from build123d import *

# Parameters (mm, degrees)
ESQUISSE1_W               = 60.5
ESQUISSE1_H               = 64
BOSS_EXTRU_1_DEPTH        = 30
ESQUISSE2_R               = 4.5
ENL_V_MAT_EXTRU_1_DEPTH   = 32
ENL_V_MAT_EXTRU_2_REACH   = 55.283
ESQUISSE4_W               = 51.1
ESQUISSE4_H               = 83.557669167
ESQUISSE5_R               = 10.5
ENL_V_MAT_EXTRU_3_DEPTH   = 2
ESQUISSE6_R               = 10
ENL_V_MAT_EXTRU_4_DEPTH   = 4.7
ESQUISSE7_W               = 47
ESQUISSE7_H               = 57
BOSS_EXTRU_2_DEPTH        = 30
ENL_V_MAT_EXTRU_5_DEPTH   = 30
ENL_V_MAT_EXTRU_6_DEPTH   = 8.25
ESQUISSE11_W              = 5
ESQUISSE11_H              = 40.5
BOSS_EXTRU_3_DEPTH        = 5
ESQUISSE12_R              = 0.5
ENL_V_MAT_EXTRU_7_DEPTH   = 15
TROU_TARAUD_M2X0_42_D     = 1.6
TROU_TARAUD_M2X0_42_DEPTH = 17
TROU_TARAUD_M2X0_42_TIP   = 0.480688495
ENL_V_MAT_EXTRU_8_REACH   = 113.72
ESQUISSE22_W              = 82.97203866
ESQUISSE22_H              = 67.875780224
ENL_V_MAT_EXTRU_10_DEPTH  = 30
ESQUISSE23_W              = 55
ESQUISSE23_H              = 5
ESQUISSE23_H_2            = 4.9
BOSS_EXTRU_4_DEPTH        = 30
ENL_V_START               = -62
ESQUISSE24_R              = 10
ENL_V_MAT_EXTRU_11_DEPTH  = 62
ENL_V_MAT_EXTRU_12_REACH  = 111.597
ESQUISSE26_R              = 10.5
ESQUISSE26_R_2            = 4.5
BOSS_EXTRU_5_DEPTH        = 5
ESQUISSE27_R              = 10.5
ENL_V_MAT_EXTRU_13_DEPTH  = 2.5
ESQUISSE28_W              = 21.53784572
ESQUISSE28_H              = 33.22443827
ENL_V_MAT_EXTRU_14_DEPTH  = 5
ESQUISSE29_W              = 5
ESQUISSE29_H              = 52.1
ENL_V_MAT_EXTRU_15_DEPTH  = 30
BOSS_EXTRU_6_DEPTH        = 62
ENL_V_START_2             = -20.388398
ESQUISSE32_W              = 38.789198293
ESQUISSE32_H              = 52.1
ENL_V_MAT_EXTRU_16_DEPTH  = 20.388398
ESQUISSE36_W              = 70.879809572
ESQUISSE36_H              = 44.299384872
ENL_V_MAT_EXTRU_20_DEPTH  = 62
ESQUISSE37_W              = 30
ESQUISSE37_H              = 4.9
ESQUISSE37_H_2            = 5
BOSS_EXTRU_8_DEPTH        = 70
ENL_V_MAT_EXTRU_21_REACH  = 119.544
ESQUISSE38_R              = 4.5
ESQUISSE39_R              = 10
ENL_V_MAT_EXTRU_22_DEPTH  = 4.9
ESQUISSE40_R              = 10.5
ENL_V_MAT_EXTRU_23_DEPTH  = 2.5
ENL_V_MAT_EXTRU_24_REACH  = 119.544


with BuildPart() as part:
    # Esquisse1 → Boss.-Extru.1 (new body)
    with BuildSketch(Plane.XY):
        Rectangle(ESQUISSE1_W, ESQUISSE1_H)
    extrude(amount=BOSS_EXTRU_1_DEPTH)

    # Esquisse2 → Enlèv. mat.-Extru.1 (cut)
    with BuildSketch(Plane(origin=(30.25, 0, 0), x_dir=(0, 0, -1), z_dir=(1, 0, 0))):
        with Locations(Location((-15, -17, 0), (0, 0, 90))):
            Circle(ESQUISSE2_R)
    extrude(amount=-ENL_V_MAT_EXTRU_1_DEPTH, mode=Mode.SUBTRACT)

    # Enlèv. mat.-Extru.2: up to this face of the body (flat: up to its plane)
    enl_v_mat_extru_2_end = Plane(part.part.faces().sort_by_distance((0, 0, 0))[0])
    # Esquisse4 → Enlèv. mat.-Extru.2 (cut, up to the picked face)
    with BuildSketch(Plane.XY.offset(30), mode=Mode.PRIVATE) as enl_v_mat_extru_2_sk1:
        with Locations((0, -14.778834584)):
            Rectangle(ESQUISSE4_W, ESQUISSE4_H)
    enl_v_mat_extru_2_tool1 = split(extrude(enl_v_mat_extru_2_sk1.sketch, amount=-ENL_V_MAT_EXTRU_2_REACH, mode=Mode.PRIVATE), bisect_by=enl_v_mat_extru_2_end, keep=Keep.BOTH, mode=Mode.PRIVATE)
    add(enl_v_mat_extru_2_tool1.solids().sort_by(Axis((0, -14.778835, 30), (0, 0, -1)))[0], mode=Mode.SUBTRACT)

    # Esquisse5 → Enlèv. mat.-Extru.3 (cut)
    with BuildSketch(Plane(origin=(30.25, 0, 0), x_dir=(0, 0, -1), z_dir=(1, 0, 0))):
        with Locations(Location((-15, -17, 0), (0, 0, 90))):
            Circle(ESQUISSE5_R)
    extrude(amount=-ENL_V_MAT_EXTRU_3_DEPTH, mode=Mode.SUBTRACT)

    # Esquisse6 → Enlèv. mat.-Extru.4 (cut)
    with BuildSketch(Plane(origin=(-25.55, 0, 0), x_dir=(0, 0, -1), z_dir=(1, 0, 0))):
        with Locations((-15, -17)):
            Circle(ESQUISSE6_R)
    extrude(amount=-ENL_V_MAT_EXTRU_4_DEPTH, mode=Mode.SUBTRACT)

    # Esquisse7 → Boss.-Extru.2 (add)
    with BuildSketch(Plane.XY.offset(30)):
        with Locations((-6.75, 60.5)):
            Rectangle(ESQUISSE7_W, ESQUISSE7_H)
    extrude(amount=-BOSS_EXTRU_2_DEPTH)

    # Esquisse8 → Enlèv. mat.-Extru.5 (cut)
    with BuildSketch(Plane.XY.offset(30)):
        Polygon((-15.25, 80.75), (11.75, 80.75), (11.75, 101.149817475), (21.75, 101.149817475), (21.75, 32), (11.75, 32), (11.75, 40.25), (-15.25, 40.25), align=None)
    extrude(amount=-ENL_V_MAT_EXTRU_5_DEPTH, mode=Mode.SUBTRACT)

    # Esquisse10 → Enlèv. mat.-Extru.6 (cut)
    with BuildSketch(Plane.XZ.offset(-80.75)):
        Polygon((-5.25, 11), (-5.25, 12), (34.75, 12), (34.75, 18), (-5.25, 18), (-5.25, 19), (-15.25, 19), (-15.25, 11), align=None)
    extrude(amount=-ENL_V_MAT_EXTRU_6_DEPTH, mode=Mode.SUBTRACT)

    # Esquisse11 → Boss.-Extru.3 (add)
    with BuildSketch(Plane(origin=(-15.25, 0, 0), x_dir=(0, 0, -1), z_dir=(1, 0, 0))):
        with Locations((-27.5, 60.5)):
            Rectangle(ESQUISSE11_W, ESQUISSE11_H)
        with Locations((-2.5, 60.5)):
            Rectangle(ESQUISSE11_W, ESQUISSE11_H)
    extrude(amount=BOSS_EXTRU_3_DEPTH)

    # Esquisse12 → Enlèv. mat.-Extru.7 (cut)
    with BuildSketch(Plane(origin=(11.75, 0, 0), x_dir=(0, 0, -1), z_dir=(1, 0, 0))):
        with Locations((-19.925, 85.21)):
            Circle(ESQUISSE12_R)
        with Locations(Location((-10.075, 85.21, 0), (0, 0, 180))):
            Circle(ESQUISSE12_R)
        with Locations((-10.075, 35.79)):
            Circle(ESQUISSE12_R)
        with Locations(Location((-19.925, 35.79, 0), (0, 0, 180))):
            Circle(ESQUISSE12_R)
    extrude(amount=-ENL_V_MAT_EXTRU_7_DEPTH, mode=Mode.SUBTRACT)

    # Trou taraudé M2x0.42
    with Locations(Plane(origin=(11.75, 85.21, 19.925), x_dir=(0, 0, 1), z_dir=(1, 0, 0))):
        with Locations((0, 0), (-9.85, 0), (-9.85, 49.42), (0, 49.42)):
            Hole(TROU_TARAUD_M2X0_42_D / 2, depth=TROU_TARAUD_M2X0_42_DEPTH)
            with Locations((0, 0, -(TROU_TARAUD_M2X0_42_DEPTH + TROU_TARAUD_M2X0_42_TIP / 2))):  # 118° drill point
                Cone(0, TROU_TARAUD_M2X0_42_D / 2, TROU_TARAUD_M2X0_42_TIP, mode=Mode.SUBTRACT)

    # Enlèv. mat.-Extru.8: up to this face of the body (flat: up to its plane)
    enl_v_mat_extru_8_end = Plane(part.part.faces().sort_by_distance((30.25, 3.741727612, 15))[0])
    # Esquisse15 → Enlèv. mat.-Extru.8 (cut, up to the picked face)
    with BuildSketch(Plane.ZY.offset(30.25), mode=Mode.PRIVATE) as enl_v_mat_extru_8_sk1:
        with BuildLine():
            Line((40, -17), (30, -17))
            ThreePointArc((30, -17), (15, -32), (0, -17))
            Line((0, -17), (-10, -17))
            ThreePointArc((-10, -17), (15, -42), (40, -17))
        make_face()
    enl_v_mat_extru_8_tool1 = split(extrude(enl_v_mat_extru_8_sk1.sketch, amount=-ENL_V_MAT_EXTRU_8_REACH, mode=Mode.PRIVATE), bisect_by=enl_v_mat_extru_8_end, keep=Keep.BOTH, mode=Mode.PRIVATE)
    add(enl_v_mat_extru_8_tool1.solids().sort_by(Axis((-30.25, -17.559017, -5), (1, 0, 0)))[0], mode=Mode.SUBTRACT)

    # Esquisse22 → Enlèv. mat.-Extru.10 (cut)
    with BuildSketch(Plane.XY.offset(30)):
        with Locations((-1.917421061, -6.937890112)):
            Rectangle(ESQUISSE22_W, ESQUISSE22_H)
    extrude(amount=-ENL_V_MAT_EXTRU_10_DEPTH, mode=Mode.SUBTRACT)

    # Esquisse23 → Boss.-Extru.4 (add)
    with BuildSketch(Plane(origin=(0, 0, 0), x_dir=(-1, 0, 0), z_dir=(0, 0, -1))):
        with Locations((57.75, 29.5)):
            Rectangle(ESQUISSE23_W, ESQUISSE23_H)
        with Locations((57.75, 86.55)):
            Rectangle(ESQUISSE23_W, ESQUISSE23_H_2)
    extrude(amount=-BOSS_EXTRU_4_DEPTH)

    # Esquisse24 → Enlèv. mat.-Extru.11 (cut)
    with BuildSketch(Plane.XZ.offset(-27).offset(ENL_V_START)):
        with Locations((-74.25, 15)):
            Circle(ESQUISSE24_R)
    extrude(amount=ENL_V_MAT_EXTRU_11_DEPTH, mode=Mode.SUBTRACT)

    # Enlèv. mat.-Extru.12: up to this face of the body (flat: up to its plane)
    enl_v_mat_extru_12_end = Plane(part.part.faces().sort_by_distance((-34.437928466, 89, 15))[0])
    # Esquisse25 → Enlèv. mat.-Extru.12 (cut, up to the picked face)
    with BuildSketch(Plane.XZ.offset(-27), mode=Mode.PRIVATE) as enl_v_mat_extru_12_sk1:
        with BuildLine():
            Line((-74.25, 44.134833893), (-74.25, 30))
            ThreePointArc((-74.25, 30), (-89.25, 15), (-74.25, 0))
            Line((-74.25, 0), (-74.25, -14.134833893))
            ThreePointArc((-74.25, -14.134833893), (-103.384833893, 15), (-74.25, 44.134833893))
        make_face()
    enl_v_mat_extru_12_tool1 = split(extrude(enl_v_mat_extru_12_sk1.sketch, amount=-ENL_V_MAT_EXTRU_12_REACH, mode=Mode.PRIVATE), bisect_by=enl_v_mat_extru_12_end, keep=Keep.BOTH, mode=Mode.PRIVATE)
    add(enl_v_mat_extru_12_tool1.solids().sort_by(Axis((-74.901475, 27, 37.067417), (0, 1, 0)))[0], mode=Mode.SUBTRACT)

    # Esquisse26 → Boss.-Extru.5 (add)
    with BuildSketch(Plane.XZ.offset(-27)):
        with Locations((-74.25, 15)):
            Circle(ESQUISSE26_R)
        with Locations((-74.25, 15)):
            Circle(ESQUISSE26_R_2, mode=Mode.SUBTRACT)
    extrude(amount=-BOSS_EXTRU_5_DEPTH)

    # Esquisse27 → Enlèv. mat.-Extru.13 (cut)
    with BuildSketch(Plane.XZ.offset(-27)):
        with Locations((-74.25, 15)):
            Circle(ESQUISSE27_R)
    extrude(amount=-ENL_V_MAT_EXTRU_13_DEPTH, mode=Mode.SUBTRACT)

    # Esquisse28 → Enlèv. mat.-Extru.14 (cut)
    with BuildSketch(Plane(origin=(0, 32, 0), x_dir=(1, 0, 0), z_dir=(0, 1, 0))):
        with Locations((22.51892286, -16.612219135)):
            Rectangle(ESQUISSE28_W, ESQUISSE28_H)
    extrude(amount=-ENL_V_MAT_EXTRU_14_DEPTH, mode=Mode.SUBTRACT)

    # Esquisse29 → Enlèv. mat.-Extru.15 (cut)
    with BuildSketch(Plane(origin=(0, 0, 0), x_dir=(-1, 0, 0), z_dir=(0, 0, -1))):
        with Locations((27.75, 58.05)):
            Rectangle(ESQUISSE29_W, ESQUISSE29_H)
    extrude(amount=-ENL_V_MAT_EXTRU_15_DEPTH, mode=Mode.SUBTRACT)

    # Esquisse31 → Boss.-Extru.6 (add)
    with BuildSketch(Plane.XZ.offset(-27)):
        with BuildLine():
            ThreePointArc((-74.826036871, 4.515812787), (-83.84709586, 10.740217019), (-82.411654216, 21.605861069))
            Line((-82.411654216, 21.605861069), (-85.25, 25.198039027))
            Line((-85.25, 25.198039027), (-85.25, 4.801960973))
            Line((-85.25, 4.801960973), (-74.826036871, 4.515812787))
        make_face()
        with BuildLine():
            ThreePointArc((-85.25, 25.198039027), (-89.25, 15), (-85.25, 4.801960973))
            Line((-85.25, 4.801960973), (-85.25, 25.198039027))
        make_face()
    extrude(amount=-BOSS_EXTRU_6_DEPTH)

    # Esquisse32 → Enlèv. mat.-Extru.16 (cut)
    with BuildSketch(Plane(origin=(0.067526976, 0, 2.459909751), x_dir=(-0.9996234341769173, 0, 0.027440660421105302), z_dir=(-0.027440660421105302, 0, -0.9996234341769173)).offset(ENL_V_START_2)):
        with Locations((94.316375975, 58.05)):
            Rectangle(ESQUISSE32_W, ESQUISSE32_H)
    extrude(amount=ENL_V_MAT_EXTRU_16_DEPTH, mode=Mode.SUBTRACT)

    # Esquisse36 → Enlèv. mat.-Extru.20 (cut)
    with BuildSketch(Plane.XZ.offset(-27)):
        with Locations((-60.689904786, 17.333529037)):
            Rectangle(ESQUISSE36_W, ESQUISSE36_H)
    extrude(amount=-ENL_V_MAT_EXTRU_20_DEPTH, mode=Mode.SUBTRACT)

    # Esquisse37 → Boss.-Extru.8 (add)
    with BuildSketch(Plane.ZY.offset(25.25)):
        with Locations((15, 86.55)):
            Rectangle(ESQUISSE37_W, ESQUISSE37_H)
        with Locations((15, 29.5)):
            Rectangle(ESQUISSE37_W, ESQUISSE37_H_2)
    extrude(amount=BOSS_EXTRU_8_DEPTH)

    # Enlèv. mat.-Extru.21: up to this face of the body (flat: up to its plane)
    enl_v_mat_extru_21_end = Plane(part.part.faces().sort_by_distance((-44.098084544, 89, 15))[0])
    # Esquisse38 → Enlèv. mat.-Extru.21 (cut, up to the picked face)
    with BuildSketch(Plane.XZ.offset(-27), mode=Mode.PRIVATE) as enl_v_mat_extru_21_sk1:
        with Locations((-80.25, 15)):
            Circle(ESQUISSE38_R)
    enl_v_mat_extru_21_tool1 = split(extrude(enl_v_mat_extru_21_sk1.sketch, amount=-ENL_V_MAT_EXTRU_21_REACH, mode=Mode.PRIVATE), bisect_by=enl_v_mat_extru_21_end, keep=Keep.BOTH, mode=Mode.PRIVATE)
    add(enl_v_mat_extru_21_tool1.solids().sort_by(Axis((-80.25, 27, 15), (0, 1, 0)))[0], mode=Mode.SUBTRACT)

    # Esquisse39 → Enlèv. mat.-Extru.22 (cut)
    with BuildSketch(Plane(origin=(0, 89, 0), x_dir=(1, 0, 0), z_dir=(0, 1, 0))):
        with Locations(Location((-80.25, -15, 0), (0, 0, 270))):
            Circle(ESQUISSE39_R)
    extrude(amount=-ENL_V_MAT_EXTRU_22_DEPTH, mode=Mode.SUBTRACT)

    # Esquisse40 → Enlèv. mat.-Extru.23 (cut)
    with BuildSketch(Plane.XZ.offset(-27)):
        with Locations((-80.25, 15)):
            Circle(ESQUISSE40_R)
    extrude(amount=-ENL_V_MAT_EXTRU_23_DEPTH, mode=Mode.SUBTRACT)

    # Enlèv. mat.-Extru.24: up to this face of the body (flat: up to its plane)
    enl_v_mat_extru_24_end = Plane(part.part.faces().sort_by_distance((-39.91307138, 89, 15))[0])
    # Esquisse42 → Enlèv. mat.-Extru.24 (cut, up to the picked face)
    with BuildSketch(Plane.XZ.offset(-27), mode=Mode.PRIVATE) as enl_v_mat_extru_24_sk1:
        with BuildLine():
            Line((-80.25, 38.922928663), (-80.25, 30))
            ThreePointArc((-80.25, 30), (-95.25, 15), (-80.25, 0))
            Line((-80.25, 0), (-80.25, -8.922928663))
            ThreePointArc((-80.25, -8.922928663), (-104.172928663, 15), (-80.25, 38.922928663))
        make_face()
    enl_v_mat_extru_24_tool1 = split(extrude(enl_v_mat_extru_24_sk1.sketch, amount=-ENL_V_MAT_EXTRU_24_REACH, mode=Mode.PRIVATE), bisect_by=enl_v_mat_extru_24_end, keep=Keep.BOTH, mode=Mode.PRIVATE)
    add(enl_v_mat_extru_24_tool1.solids().sort_by(Axis((-80.784933, 27, 34.461464), (0, 1, 0)))[0], mode=Mode.SUBTRACT)


solid = part.part
Verification items for the finished model (mm, model axes). A direction names the side the tool comes from. Coordinates: 2 decimals unless noted, no trailing zeros. Order: outer loops, then holes, each group sorted by start corner. A loop starts at its lowest first (then second) coordinate and runs counter-clockwise, first axis right, second up.
Item 1: Depth check by flat-ended pin: pin 1 (1.4 mm diameter, centred on y = 35.79, z = 10.075, fed in from +X); pin 2 (2.5 mm diameter, centred on y = 85.21, z = 19.925, fed in from -X); pin 3 (12 mm diameter, centred on x = -84, y = 77, fed in from -Z); pin 4 (2.5 mm diameter, centred on y = 51, z = 28, fed in from +X). Enter the tip coordinate at first touch or a pass-through.
Filled in:
pin 1: stops at x = -5.31
pin 2: stops at x = -94.79
pin 3: passes through
pin 4: stops at x = -10.25
Item 2: Release check for a two-part mould opening along X. For faces 1 (the face through (-10.25, 61, 28)), 2 (the face through (-2, 40.25, 15)), 3 (the face through (-84.746, 30.732, 15.198)) record: +X half, -X half, draft (parallel to the pull), parting line (faces both ways), or undercut.
Filled in:
face 1: +X half
face 2: draft
face 3: undercut
Item 3: Material ranges on L1, parallel to Z at x = 0.5, y = 35.79 (3 decimals); L2, parallel to Z at x = 3.75, y = 85.21 (3 decimals); L3, parallel to Z at x = -10.5, y = 44.5, recorded low to high.
Filled in:
L1: z = 0 to 9.275, 10.875 to 19.125, 20.725 to 30
L2: z = 0 to 9.275, 10.875 to 12, 18 to 19.125, 20.725 to 30
L3: z = 0 to 5, 25 to 30
Item 4: Section check A-A, the plane z = 15. Enter the section's corners in (x, y), then the cut area to 3 significant figures.
Filled in:
outline: (-95.25, 27) - (-90.75, 27) - (-90.75, 29.5) - (-84.75, 29.5) - (-84.75, 32) - (-95.25, 32) - close; (-95.25, 84.1) - (-90.25, 84.1) - (-90.25, 89) - (-95.25, 89) - close; (-75.75, 29.5) - (-69.75, 29.5) - (-69.75, 27) - (11.75, 27) - (11.75, 40.25) - (-15.25, 40.25) - (-15.25, 89) - (-70.25, 89) - (-70.25, 84.1) - (-25.25, 84.1) - (-25.25, 32) - (-75.75, 32) - close
area: 1,500 mm2
Item 5: Section check B-B, the plane x = -47. Enter the section's corners in (y, z), then the cut area to 3 significant figures.
Filled in:
outline: (27, 0) - (32, 0) - (32, 30) - (27, 30) - close; (84.1, 0) - (89, 0) - (89, 30) - (84.1, 30) - close
area: 297 mm2
Item 6: Access from +Z, -Z, +X, -X, +Y, -Y to the whole of each face (thin tool, end or side, straight path). Record for faces 4 (the face through (3, 85, 18)), 5 (the face through (-10, 85, 19)), 6 (the face through (-25.25, 58, 15)), 7 (the face through (-10.25, 61, 3)).
Filled in:
face 4: +X, +Y
face 5: +Y
face 6: +Z, -Z, -X
face 7: +Z, -Z, +X
